Source: CAD feature listing. Evaluate the final solid. Frame: model axes, mm. Face numbers are marked on the shaded views. A direction names the side the tool comes from. Give positions to 0.01 mm unless a question says otherwise; leave off trailing zeros. Loops run counter-clockwise (first coordinate to the right, second up) from the corner with the lowest first, then second, coordinate; pieces in that order, holes last. Notation, with made-up numbers: M 22,-20 L 59,-20 A25 ccw 59,15 Z; hole C 2,-10 d11. An arc over 180 degrees is marked long. Put each result on its own line as item: value.
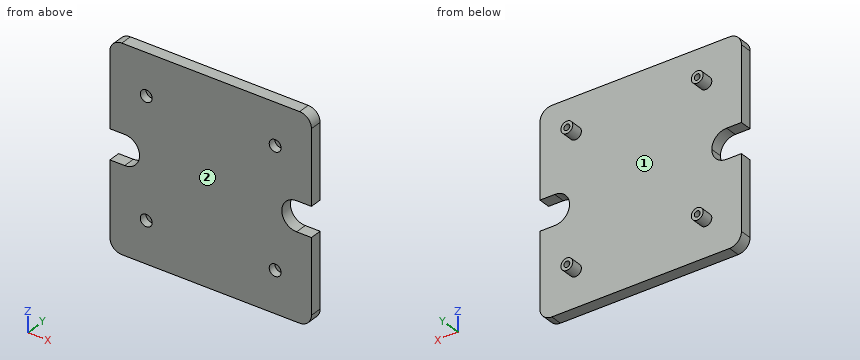
from build123d import *

# Parameters (mm, degrees)
SKETCH2_W           = 170
SKETCH2_H           = 170
BOSS_EXTRUDE1_DEPTH = 10
SKETCH1_R           = 5
SKETCH1_R_2         = 2.5
BOSS_EXTRUDE2_DEPTH = 20
FILLET1_R           = 10
SKETCH3_R           = 5
CUT_EXTRUDE1_DEPTH  = 6.5
CUT_EXTRUDE2_DEPTH  = 11


with BuildPart() as part:
    # Sketch2 → Boss-Extrude1 (new body)
    with BuildSketch(Plane(origin=(0, 0, 0), x_dir=(1, 0, 0), z_dir=(0, 1, 0))):
        with Locations((85, 85)):
            Rectangle(SKETCH2_W, SKETCH2_H)
    extrude(amount=BOSS_EXTRUDE1_DEPTH)

    # Sketch1 → Boss-Extrude2 (add)
    with BuildSketch(Plane(origin=(0, 0, 0), x_dir=(1, 0, 0), z_dir=(0, 1, 0))):
        with Locations((30, 30)):
            Circle(SKETCH1_R)
        with Locations((30, 30)):
            Circle(SKETCH1_R_2, mode=Mode.SUBTRACT)
        with Locations((140, 30)):
            Circle(SKETCH1_R)
        with Locations((140, 30)):
            Circle(SKETCH1_R_2, mode=Mode.SUBTRACT)
        with Locations((30, 140)):
            Circle(SKETCH1_R)
        with Locations((30, 140)):
            Circle(SKETCH1_R_2, mode=Mode.SUBTRACT)
        with Locations((140, 140)):
            Circle(SKETCH1_R)
        with Locations((140, 140)):
            Circle(SKETCH1_R_2, mode=Mode.SUBTRACT)
    extrude(amount=BOSS_EXTRUDE2_DEPTH)

    # Fillet1
    fillet1_edges = [part.edges().sort_by_distance(p)[0] for p in [
        (0, 5, -170),
        (170, 5, -170),
        (170, 5, 0),
        (0, 5, 0),
    ]]
    fillet(fillet1_edges, radius=FILLET1_R)

    # Sketch3 → Cut-Extrude1 (cut)
    with BuildSketch(Plane(origin=(0, 0, 0), x_dir=(-1, 0, 0), z_dir=(0, -1, 0))):
        with Locations((-30.625, 135)):
            Circle(SKETCH3_R)
        with Locations((-139.375, 135)):
            Circle(SKETCH3_R)
        with Locations((-139.375, 35)):
            Circle(SKETCH3_R)
        with Locations((-30.625, 35)):
            Circle(SKETCH3_R)
    extrude(amount=-CUT_EXTRUDE1_DEPTH, mode=Mode.SUBTRACT)

    # Sketch4 → Cut-Extrude2 (cut, through all)
    with BuildSketch(Plane(origin=(0, 10, 0), x_dir=(1, 0, 0), z_dir=(0, 1, 0))):
        with BuildLine():
            ThreePointArc((25, 85), (21.338834765, 93.838834765), (12.5, 97.5))
            Line((12.5, 97.5), (0, 97.5))
            Line((0, 97.5), (0, 72.5))
            Line((0, 72.5), (12.5, 72.5))
            ThreePointArc((12.5, 72.5), (21.338834765, 76.161165235), (25, 85))
        make_face()
        with BuildLine():
            ThreePointArc((157.5, 97.5), (145, 85), (157.5, 72.5))
            Line((157.5, 72.5), (170, 72.5))
            Line((170, 72.5), (170, 97.5))
            Line((170, 97.5), (157.5, 97.5))
        make_face()
    extrude(amount=-CUT_EXTRUDE2_DEPTH, mode=Mode.SUBTRACT)


solid = part.part
1. Section query A-A (y = 14). Output: boundary loops of the cut face in (x, z), plus the area to 3 significant figures.
Found:
outline: C 30,-140 d10; C 30,-30 d10; C 140,-140 d10; C 140,-30 d10; hole C 30,-140 d5; hole C 30,-30 d5; hole C 140,-140 d5; hole C 140,-30 d5
area: 236 mm^2
2. Material intervals for line 1 (X direction, y = 14.5, z = -140); line 2 (Z direction, x = 140, y = 12.75); line 3 (X direction, y = 2.75, z = -135) (3 decimals), sorted ascending. Write a range as from..to.
Found:
line 1: 25..27.5, 32.5..35, 135..137.5, 142.5..145
line 2: -145..-142.5, -137.5..-135, -35..-32.5, -27.5..-25
line 3: 0..25.625, 35.625..134.375, 144.375..170
3. Section query C-C (z = -64). Output: boundary loops of the cut face in (x, y).
Found:
outline: M 0,0 L 170,0 L 170,10 L 0,10 Z
4. Section query B-B (y = 4). Output: boundary loops of the cut face in (x, z) (3 decimals).
Found:
outline: M 0,-160 A10 ccw 10,-170 L 160,-170 A10 ccw 170,-160 L 170,-97.5 L 157.5,-97.5 A12.5 cw 157.5,-72.5 L 170,-72.5 L 170,-10 A10 ccw 160,0 L 10,0 A10 ccw 0,-10 L 0,-72.5 L 12.5,-72.5 A12.5 cw 12.5,-97.5 L 0,-97.5 Z; hole C 30.625,-135 d10; hole C 30.625,-35 d10; hole C 139.375,-135 d10; hole C 139.375,-35 d10
5. Contact query for flat-ended pins moving along their axis: P1, Ø5, axis at x = 32.5, z = -136.5, coming from the -Y side; P2, Ø5, axis at x = 5.5, y = 3.5, coming from the -Z side; P3, Ø2.5, axis at x = 139.5, z = -140.5, coming from the +Y side. Output: stop coordinate, or through.
Found:
P1: y = 6.5
P2: z = -169.8
P3: y = 10
6. Access query for the marked faces 1 and 2. Directions: +Z, -Z, +X, -X, +Y, -Y. A direction counts if a zero-diameter tool reaches every point of the face in a straight line with its end or side. Return the directions, or none.
Found:
face 1: +Y
face 2: +Z, -Z, +X, -X, -Y
7. Section query D-D (x = 30). Output: boundary loops of the cut face in (y, z).
Found:
outline: M 0,-170 L 10,-170 L 10,-145 L 20,-145 L 20,-142.5 L 10,-142.5 L 10,-137.5 L 20,-137.5 L 20,-135 L 10,-135 L 10,-35 L 20,-35 L 20,-32.5 L 10,-32.5 L 10,-27.5 L 20,-27.5 L 20,-25 L 10,-25 L 10,0 L 0,0 L 0,-30.04 L 6.5,-30.04 L 6.5,-39.96 L 0,-39.96 L 0,-130.04 L 6.5,-130.04 L 6.5,-139.96 L 0,-139.96 Z
